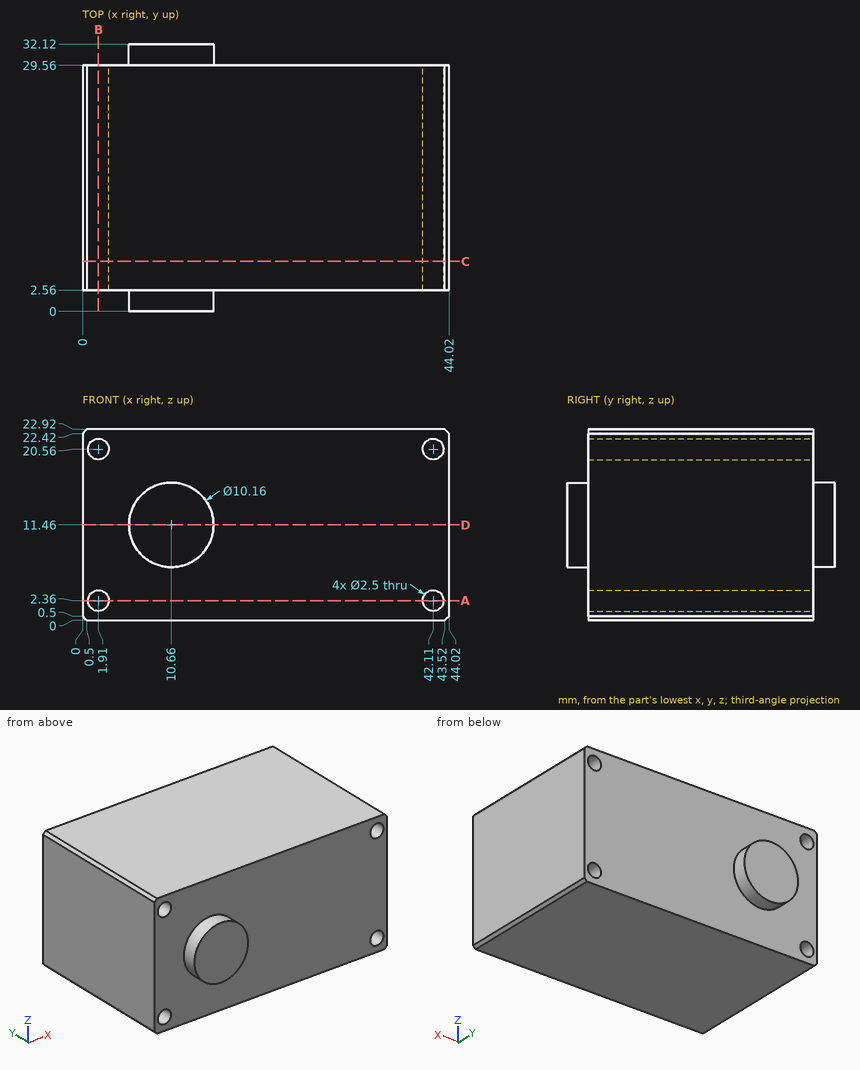
Design review of the part shown in the three views and the two pictorial views. Dimensions are in mm from the part's minimum x, y and z. Give positions to 0.01 mm unless a question says otherwise; leave off trailing zeros. Loops run counter-clockwise (first coordinate to the right, second up) from the corner with the lowest first, then second, coordinate; pieces in that order, holes last. Notation, with made-up numbers: M 82,-40 L 86,-40 A22 ccw 86,-7 Z; hole C 45,27.25 d7. An arc over 180 degrees is marked long. Put each result on its own line as item: value. Start each with the question number.
(1) Add section D-D, the plane z = 11.46. Write out the cut boundary in (x, y).
(2) For pin 1 (1 mm diameter, centred on x = 16, z = 7.5, fed in from +Y); pin 2 (12 mm diameter, centred on x = 12, y = 24.5, fed in from -Z); pin 3 (3 mm diameter, centred on x = 1.91, z = 2.36, fed in from -Y); pin 4 (2 mm diameter, centred on x = 42.11, z = 2.36, fed in from -Y), all flat-tipped, find the tip position at first contact; note any pin that passes through.
(3) Add section C-C, the plane y = 6. Write out the cut boundary in (x, z), then the cut area to 3 significant figures.
(4) Add section B-B, the plane x = 1.91. Write out the cut boundary in (y, z), then the cut area to 3 significant figures.
(5) Wall thickness on L1, parallel to X at y = 19.75, z = 20.56; L2, parallel to Z at x = 42.11, y = 12; L3, parallel to Z at x = 1, y = 23: over which ranges is each line inside the solid? List them lowest first.
(6) Add section A-A, the plane z = 2.36. Write out the cut boundary in (x, y), then the cut area to 3 significant figures.
Result:
1. outline: M 0,2.56 L 5.58,2.56 L 5.58,0 L 15.74,0 L 15.74,2.56 L 44.02,2.56 L 44.02,29.56 L 15.74,29.56 L 15.74,32.12 L 5.58,32.12 L 5.58,29.56 L 0,29.56 Z
2. pin 1: stops at y = 29.56
2. pin 2: stops at z = 0
2. pin 3: stops at y = 2.56
2. pin 4: passes through
3. outline: M 0,0.5 L 0.5,0 L 43.52,0 L 44.02,0.5 L 44.02,22.42 L 43.52,22.92 L 0.5,22.92 L 0,22.42 Z; hole C 1.91,2.36 d2.5; hole C 1.91,20.56 d2.5; hole C 42.11,2.36 d2.5; hole C 42.11,20.56 d2.5
3. area: 989 mm^2
4. outline: M 2.56,0 L 29.56,0 L 29.56,1.11 L 2.56,1.11 Z; M 2.56,3.61 L 29.56,3.61 L 29.56,19.31 L 2.56,19.31 Z; M 2.56,21.81 L 29.56,21.81 L 29.56,22.92 L 2.56,22.92 Z
4. area: 484 mm^2
5. L1: x = 0 to 0.66, 3.16 to 40.86, 43.36 to 44.02
5. L2: z = 0 to 1.11, 3.61 to 19.31, 21.81 to 22.92
5. L3: z = 0 to 1.5, 3.22 to 19.7, 21.42 to 22.92
6. outline: M 0,2.56 L 0.66,2.56 L 0.66,29.56 L 0,29.56 Z; M 3.16,2.56 L 40.86,2.56 L 40.86,29.56 L 3.16,29.56 Z; M 43.36,2.56 L 44.02,2.56 L 44.02,29.56 L 43.36,29.56 Z
6. area: 1,050 mm^2
